For this review, take the finished solid that the model builds, in its own axes (mm). A direction names the side the tool comes from. Give positions to 0.01 mm unless a question says otherwise; leave off trailing zeros. Write each loop counter-clockwise with the first axis right and the second up, starting at its lowest first coordinate (ties: lowest second). Pieces come first, ordered by that corner, then holes. Notation, with made-up numbers: (72, 57) -> (131, 57) arc R23 cw to (131, 66) -> close; hole circle Ø5 at (61, 26). An arc over 180 degrees is marked (long way). Answer as CSV lines item,"result".
```python
from build123d import *

# Parameters (mm, degrees)
F0_W      = 25
F0_H      = 11
F1_DEPTH  = 10
F2_R      = 8
F3_DEPTH  = 6
F4_R      = 6
F5_DEPTH  = 6
F6_W      = 11
F6_H      = 10
F7_DEPTH  = 2
F8_W      = 11
F8_H      = 10
F9_DEPTH  = 2
F10_R     = 1.75
F11_DEPTH = 25


with BuildPart() as f1:
    # F0 (on Top) → F1 (new body)
    with BuildSketch(Plane.XY):
        with Locations((12.5, 5.5)):
            Rectangle(F0_W, F0_H)
    extrude(amount=F1_DEPTH)

    # F2 (on face) → F3 (cut)
    with BuildSketch(Plane.XZ):
        with Locations((12.5, 10)):
            Circle(F2_R)
    extrude(amount=-F3_DEPTH, mode=Mode.SUBTRACT)

    # F4 (on face) → F5 (cut)
    with BuildSketch(Plane(origin=(0, 11, 0), x_dir=(-1, 0, 0), z_dir=(0, 1, 0))):
        with Locations((-12.5, 10)):
            Circle(F4_R)
    extrude(amount=-F5_DEPTH, mode=Mode.SUBTRACT)

    # F6 (on face) → F7 (join)
    with BuildSketch(Plane(origin=(0, 0, 0), x_dir=(0, -1, 0), z_dir=(-1, 0, 0))):
        with Locations((-5.5, 5)):
            Rectangle(F6_W, F6_H)
    extrude(amount=F7_DEPTH)

    # F8 (on face) → F9 (join)
    with BuildSketch(Plane.YZ.offset(25)):
        with Locations((5.5, 5)):
            Rectangle(F8_W, F8_H)
    extrude(amount=F9_DEPTH)

    # F10 (on face) → F11 (cut)
    with BuildSketch(Plane.XY.offset(10)):
        with Locations((0.75, 6.25)):
            Circle(F10_R)
        with Locations((24.25, 6.25)):
            Circle(F10_R)
    extrude(amount=-F11_DEPTH, mode=Mode.SUBTRACT)


solid = f1.part
```
Q1. Add section D-D (z = 5.5). Write out the cut boundary in (x, y), plus the area to 3 significant figures.
Answer block:
outline,"(-2, 0) -> (5.89, 0) -> (5.89, 6) -> (8.53, 6) -> (8.53, 11) -> (-2, 11) -> close; (16.47, 6) -> (19.11, 6) -> (19.11, 0) -> (27, 0) -> (27, 11) -> (16.47, 11) -> close; hole circle Ø3.5 at (0.75, 6.25); hole circle Ø3.5 at (24.25, 6.25)"
area,"181 mm2"
Q2. Add section C-C (y = 5). Write out the cut boundary in (x, z).
Answer block:
outline,"(-2, 0) -> (-0.47, 0) -> (-0.47, 10) -> (-2, 10) -> close; (1.97, 0) -> (23.03, 0) -> (23.03, 10) -> (20.5, 10) arc R8 cw to (4.5, 10) -> (1.97, 10) -> close; (25.47, 0) -> (27, 0) -> (27, 10) -> (25.47, 10) -> close"
Q3. Draft analysis for pull direction Y (two halves, no side actions). For faces 3 (the cylindrical face through (22.86, 5.19, 5.07)), 4 (the flat face through (12.3, 11, 3.8)), 5 (the flat face through (27, 5, 5)), 6 (the cylindrical face through (0.37, 4.54, 5.07)), state which applies: released by +Y, released by -Y, zero draft, split by the parting line, or undercut.
Answer block:
face 3,"undercut"
face 4,"released by +Y"
face 5,"zero draft"
face 6,"undercut"
Q4. For faces 1 (the flat face through (11, 6, 4)), 2 (the flat face through (-2, 6, 5)), list the 3-axis set-ups (+Z, -Z, +X, -X, +Y, -Y) from which the entire face can be reached by the end or side of a thin tool; tool diameter is ignored.
Answer block:
face 1,"+Z, -Y"
face 2,"+Z, -Z, -X, +Y, -Y"
Q5. To check wall thickness, follow probe 1 along X at (y, z) = (5.5, 5) (3 decimals); probe 2 along Y at (x, z) = (0.75, 7.5); probe 3 along X at (y, z) = (6.75, 1.25). State the ranges of each line that lie inside material, in increasing order. Write a range as [from, to].
Answer block:
probe 1,"x = [-2, -0.831], [2.331, 6.255], [18.745, 22.669], [25.831, 27]"
probe 2,"y = [0, 4.5], [8, 11]"
probe 3,"x = [-2, -0.93], [2.43, 22.57], [25.93, 27]"
Q6. Add section A-A (x = 0.75). Write out the cut boundary in (y, z), plus the area to 3 significant figures.
Answer block:
outline,"(0, 0) -> (4.5, 0) -> (4.5, 10) -> (0, 10) -> close; (8, 0) -> (11, 0) -> (11, 10) -> (8, 10) -> close"
area,"75.0 mm2"
Q7. Add section B-B (z = 7.75). Write out the cut boundary in (x, y).
Answer block:
outline,"(-2, 0) -> (4.82, 0) -> (4.82, 6) -> (6.94, 6) -> (6.94, 11) -> (-2, 11) -> close; (18.06, 6) -> (20.18, 6) -> (20.18, 0) -> (27, 0) -> (27, 11) -> (18.06, 11) -> close; hole circle Ø3.5 at (0.75, 6.25); hole circle Ø3.5 at (24.25, 6.25)"
